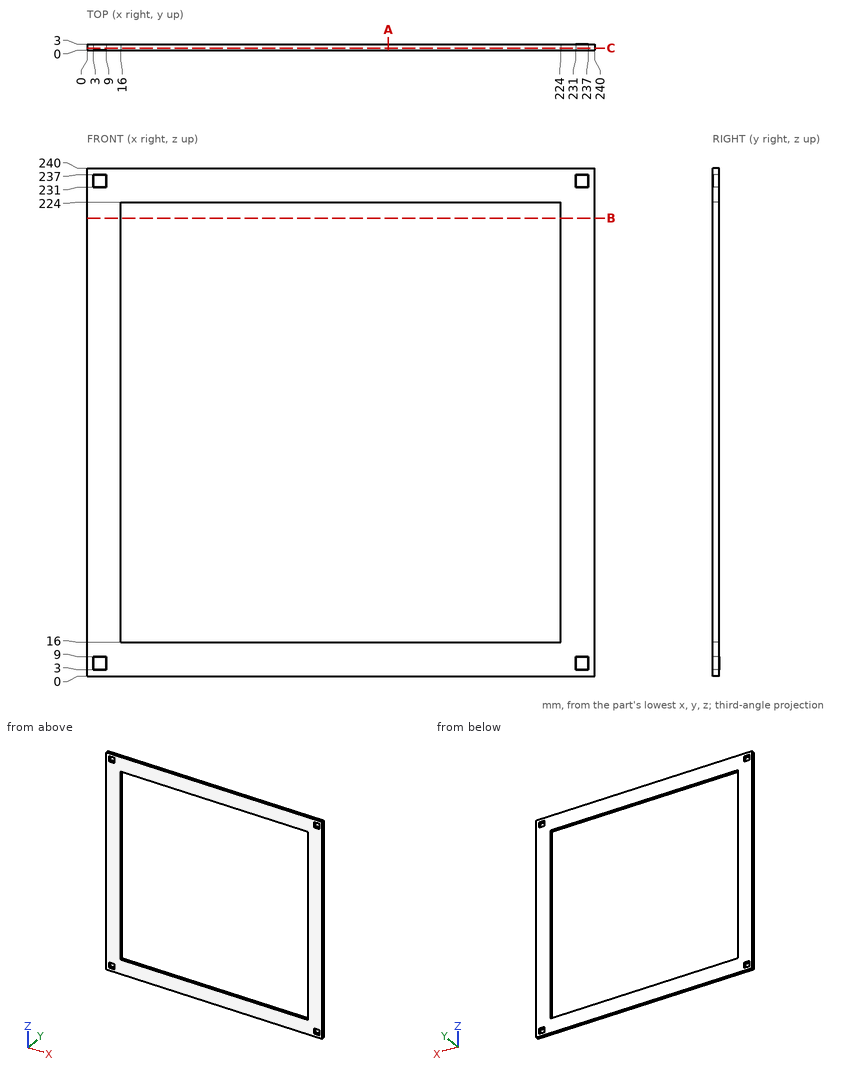
Verification items for this drawing (mm, ordinates from the low corner). Coordinates: 2 decimals unless noted, no trailing zeros. Order: outer loops, then holes, each group sorted by start corner. A loop starts at its lowest first (then second) coordinate and runs counter-clockwise, first axis right, second up. Notation, with made-up numbers: (17, 3) - (40, 3) arc R16 cw to (40, 7) - close; hole circle Ø10 at (42.5, -1). An arc over 180 degrees is marked (long way). Answer as a JSON object with one key per item and string values. Group by question number.
Item 1: Scan line: probe 1 along Z at (x, y) = (170, 0.3). Record every from-to range of solid material in increasing order.
Item 2: Sectioned sample at C-C, the plane y = 1. Record the cut outline in (x, z), and give its area (3 significant figures).
Item 3: Sectioned sample at B-B, the plane z = 216.5. Record the cut outline in (x, y).
Item 4: Sectioned sample at A-A, the plane x = 142.5. Record the cut outline in (y, z).
Item 5: Depth check by flat-ended pin: pin 1 Ø0.9 at (x, y) = (142, 1) entering from -Z. Enter the tip coordinate at first touch or a pass-through.
Resolved:
{
 "1": {"probe 1": "0 to 16, 224 to 240"},
 "2": {"outline": "(0, 0) - (240, 0) - (240, 240) - (0, 240) - close; hole (3, 3) - (9, 3) - (9, 9) - (3, 9) - close; hole (3, 231) - (9, 231) - (9, 237) - (3, 237) - close; hole (16, 16) - (224, 16) - (224, 224) - (16, 224) - close; hole (231, 3) - (237, 3) - (237, 9) - (231, 9) - close; hole (231, 231) - (237, 231) - (237, 237) - (231, 237) - close", "area": "14,200 mm^2"},
 "3": {"outline": "(0, 0) - (16, 0) - (16, 3) - (0, 3) - close; (224, 0) - (240, 0) - (240, 3) - (224, 3) - close"},
 "4": {"outline": "(0, 0) - (3, 0) - (3, 16) - (0, 16) - close; (0, 224) - (3, 224) - (3, 240) - (0, 240) - close"},
 "5": {"pin 1": "z = 0"}
}
